Build history of the part. All positions in model axes, mm. A direction names the side the tool comes from. Give positions to 0.01 mm unless a question says otherwise; leave off trailing zeros. Order: outer loops, then holes, each group sorted by start corner. A loop starts at its lowest first (then second) coordinate and runs counter-clockwise, first axis right, second up. Notation, with made-up numbers: (14, 81) -> (40, 81) arc R18 ccw to (40, 109) -> close; hole circle Ø7 at (35.25, -39). An arc over 180 degrees is marked (long way). Write item = value, one per line. Start each with the question number.
from build123d import *

# Parameters (mm, degrees)
F1_DEPTH = 10
F2_W     = 50
F2_H     = 3
F3_DEPTH = 25


with BuildPart() as f1:
    # F0 (on Top) → F1 (new body)
    with BuildSketch(Plane.XY):
        Polygon((-32.9432, 22.939983), (-32.935701, 19.939983), (-22.935701, 19.939983), (-22.935701, 14.939983), (-32.935701, 14.939983), (-32.935701, 11.939982), (-22.935701, 11.939982), (-22.935701, -10.060017), (27.064299, -10.060017), (27.064299, 14.939983), (-19.9357, 14.939983), (-19.9357, 16.371092), (-19.9357, 22.939983), align=None)
    extrude(amount=F1_DEPTH)

    # F2 (on face) → F3 (join)
    with BuildSketch(Plane(origin=(0, 0, 0), x_dir=(1, 0, 0), z_dir=(0, 0, -1))):
        Polygon((27.064299, -11.939983), (-22.935701, -11.939983), (-22.935701, -14.939983), (-19.9357, -14.939983), (27.064299, -14.939983), align=None)
        with Locations((2.064299, 8.560017)):
            Rectangle(F2_W, F2_H)
    extrude(amount=F3_DEPTH)


solid = f1.part
(1) Wall check: line 1 (Y direction, x = 10, z = -22); line 2 (X direction, y = 20, z = 0.5); line 3 (Z direction, x = -21.5, y = 19.5). Give the ranges that are in metal, low to high. Write a range as [from, to].
(2) Cut at C-C, the plane z = 5. Give the cut face in (x, y).
(3) Mould opens along Y. For faces 1 (the face through (-26, 22.94, 5)), 2 (the face through (2, -9, -25)), 3 (the face through (-28, 14.94, 5)) say: released by +Y, released by -Y, zero draft, split by the parting line, or undercut.
(4) 3-axis set-ups, long thin cutter, end or side, ignore diameter. For faces 4 (the face through (-19.936, 19, 5)), 5 (the face through (-22.936, 13, -12)), 6 (the face through (-28, 19.94, 5)), 7 (the face through (-22.936, -1, 4)), 8 (the face through (2, 11.94, -12)): which of +Z, -Z, +X, -X, +Y, -Y reach the whole face in a straight line?
(5) Cut at B-B, the plane x = 21.5. Give the cut face in (y, z).
(6) Cut at D-D, the plane y = 6. Give the cut face in (x, z), plus the area to 3 significant figures.
(7) Cut at A-A, the plane z = -18. Give the cut face in (x, y), plus the area to 3 significant figures.
(8) Flat gauge pins, fed straight in: P1, Ø12, axis at x = -14, z = -17.5, coming from the +Y side; P2, Ø9, axis at x = -25, y = 20.5, coming from the -Z side; P3, Ø1.5, axis at y = 13, z = 7, coming from the -X side; P4, Ø8, axis at y = 6.5, z = -18.5, coming from the -X side. Where does each tip first touch, or does it go through?
Results:
q1.line_1 = [-10.06, -7.06], [11.94, 14.94]
q1.line_2 = [-32.94, -19.94]
q1.line_3 = [0, 10]
q2.outline = (-32.94, 11.94) -> (-22.94, 11.94) -> (-22.94, -10.06) -> (27.06, -10.06) -> (27.06, 14.94) -> (-19.94, 14.94) -> (-19.94, 22.94) -> (-32.94, 22.94) -> (-32.94, 19.94) -> (-22.94, 19.94) -> (-22.94, 14.94) -> (-32.94, 14.94) -> close
q3.face_1 = released by +Y
q3.face_2 = zero draft
q3.face_3 = undercut
q4.face_4 = +Z, -Z, +X, +Y
q4.face_5 = -Z, -X, +Y, -Y
q4.face_6 = +Z, -Z, -X
q4.face_7 = +Z, -Z, -X, -Y
q4.face_8 = -Z, +X, -X
q5.outline = (-10.06, -25) -> (-7.06, -25) -> (-7.06, 0) -> (11.94, 0) -> (11.94, -25) -> (14.94, -25) -> (14.94, 10) -> (-10.06, 10) -> close
q6.outline = (-22.94, 0) -> (27.06, 0) -> (27.06, 10) -> (-22.94, 10) -> close
q6.area = 500 mm2
q7.outline = (-22.94, -10.06) -> (27.06, -10.06) -> (27.06, -7.06) -> (-22.94, -7.06) -> close; (-22.94, 11.94) -> (27.06, 11.94) -> (27.06, 14.94) -> (-22.94, 14.94) -> close
q7.area = 300 mm2
q8.P1 = 14.94
q8.P2 = 0
q8.P3 = -32.94
q8.P4 = through
